Autodesk Inventor part; units mm, degrees
ref_plane "YZ Plane" through (0, 0, 0) normal (1, 0, 0) x (0, 1, 0)
ref_plane "XZ Plane" through (0, 0, 0) normal (0, 1, 0) x (-1, 0, 0)
ref_plane "XY Plane" through (0, 0, 0) normal (0, 0, 1) x (1, 0, 0)
sketch "Sketch1" plane through (0, 0, 0) normal (0, 0, 1) x (1, 0, 0)
  line L0 (-66.5, 0) -> (-103.5, 0)
  line L1 (-103.5, 0) -> (-103.5, 18)
  line L2 (-103.5, 18) -> (-66.5, 18)
  line L3 (-66.5, 18) -> (-66.5, 0)
  line L4 (0, -3.6) -> (0, 21.6)
  point P0 (0, 0)
  dimension "d0" = 66.5
  dimension "d1" = 103.5
  dimension "d2" = 18
revolve "Revolution1" add sketch "Sketch1" angle 360 about axis through (0, -10, 0) along (0, 1, 0)
sketch "Sketch2" plane through (0, 18, 0) normal (0, 1, 0) x (1, 0, 0)
  point P0 (0, 0)
  point P1 (0, 91)
  dimension "d4" = 91
hole "Hole1" at (0, 18, -91) direction (0, -1, 0) diameter 12 end through all
pattern_circular "Circular Pattern1" count 8 over 360 about axis through (0, 9, 0) along (0, 1, 0) of "Hole1"
properties part number "CollarRingBottom" material "Stainless Steel"
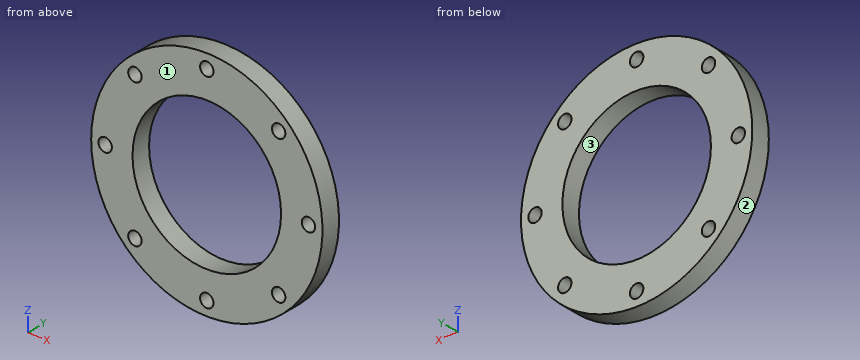
Can you work these out from the model? Positions are in its coordinate system, mm. Face numbers are marked on the shaded views. Coordinates: 2 decimals unless noted, no trailing zeros. Loops run counter-clockwise (first coordinate to the right, second up) from the corner with the lowest first, then second, coordinate; pieces in that order, holes last. Notation, with made-up numbers: (27, 72.25) - (62, 72.25) arc R22 cw to (62, 106.25) - close; hole circle Ø8 at (47, 31.25). An arc over 180 degrees is marked (long way). Answer as a JSON object with one key per item and string values. Group by question number.
Item 1: If we section it at A-A (z = 0): List the corners of the cut face in (x, y) for me.
Item 2: If we section it at D-D (x = 55): List the corners of the cut face in (y, z) for me, plus the area to 3 significant figures.
Item 3: If we section it at C-C (y = 9): State how many separate pieces and enclosed holes the cut face has, plus the area to 3 significant figures.
Item 4: If we section it at B-B (x = 0): List the corners of the cut face in (y, z) for me.
Item 5: If we mould it in two halves opening along X, with no side actions, what happens to the marked faces 1, 2 and 3? For each: released by +X, released by -X, zero draft, split by the parting line, or undercut.
Item 6: If I drill on L1, parallel to Z at x = -59.5, y = 17; L2, parallel to Z at x = 91, y = 8.5, over which ranges is the centre line in solid material (lowest first)? Write a range as from..to.
Item 7: For pin 1 (10 mm diameter, centred on y = 3, z = 51, fed in from -X); pin 2 (6 mm diameter, centred on y = 7.5, z = 46.5, fed in from -X); pin 3 (5 mm diameter, centred on x = 79, y = 10.5, fed in from -Z), each with a flat end and sliding along its axis, tell me the tip position at first contact or that it passes through.
Returned:
{
 "1": {"outline": "(-103.5, 0) - (-97, 0) - (-97, 18) - (-103.5, 18) - close; (-85, 0) - (-66.5, 0) - (-66.5, 18) - (-85, 18) - close; (66.5, 0) - (85, 0) - (85, 18) - (66.5, 18) - close; (97, 0) - (103.5, 0) - (103.5, 18) - (97, 18) - close"},
 "2": {"outline": "(0, -87.68) - (18, -87.68) - (18, -37.38) - (0, -37.38) - close; (0, 37.38) - (18, 37.38) - (18, 87.68) - (0, 87.68) - close", "area": "1,810 mm²"},
 "3": {"separate pieces": "1", "enclosed holes": "9", "area": "18,900 mm²"},
 "4": {"outline": "(0, -103.5) - (18, -103.5) - (18, -97) - (0, -97) - close; (0, -85) - (18, -85) - (18, -66.5) - (0, -66.5) - close; (0, 66.5) - (18, 66.5) - (18, 85) - (0, 85) - close; (0, 97) - (18, 97) - (18, 103.5) - (0, 103.5) - close"},
 "5": {"face 1": "zero draft", "face 2": "split by the parting line", "face 3": "undercut"},
 "6": {"L1": "z = -84.69..-67.88, -60.81..-29.7, 29.7..60.81, 67.88..84.69", "L2": "z = -49.31..-6, 6..49.31"},
 "7": {"pin 1": "stops at x = -92.72", "pin 2": "stops at x = -93.91", "pin 3": "stops at z = -69.71"}
}
